Verification items for the finished model (mm, model axes). Give positions to 0.01 mm unless a question says otherwise; leave off trailing zeros. Loops run counter-clockwise (first coordinate to the right, second up) from the corner with the lowest first, then second, coordinate; pieces in that order, holes last. Notation, with made-up numbers: (83.5, -1) -> (91.5, -1) arc R11 ccw to (91.5, 17) -> close; hole circle Ø6 at (-17.5, -33). An arc over 180 degrees is marked (long way). Answer in a Markdown table with one row per item. Add a question column.
Q1. Gauge pin test, flat ends, axial feed: P1, Ø1, axis at x = -84.5, z = 151, coming from the +Y side; P2, Ø8, axis at x = -62.5, y = 32, coming from the -Z side. Record the tip position at first contact, or that the pin passes through.
Q2. Section check C-C on y = 187.5. Give the number of separate pieces and of enclosed holes in the cut face, and give its area (3 significant figures).
Q3. Section check A-A on x = -79.5. Enter the section's corners in (y, z).
Q4. Release check for a two-part mould opening along Z. For faces 1 (the face through (-2, 6.35, 88)), 2 (the face through (2, -6.35, 88)), 3 (the face through (1, 69, 0)) record: pulls with the +Z half, pulls with the -Z half, needs draft (parallel to the pull), parting line crosses it, or undercut.
Q5. Section check B-B on z = 105.5. Enter the section's corners in (x, y), and give its area (3 significant figures).
Q6. Material ranges on probe 1 along Y at (x, z) = (0, 173); probe 2 along Z at (x, y) = (1.5, 133); probe 3 along Y at (x, z) = (38.5, 35.5), recorded low to high.
```python
from build123d import *

# Parameters (mm, degrees)
SKETCH2_W           = 38.1
SKETCH2_H           = 12.7
BOSS_EXTRUDE1_DEPTH = 12.7
SKETCH4_W           = 228.702019181
SKETCH4_H           = 12.7
BOSS_EXTRUDE2_DEPTH = 152.4
SKETCH5_R           = 25.4
BOSS_EXTRUDE3_DEPTH = 12.7


with BuildPart() as part:
    # Sketch2 → Boss-Extrude1 (new body)
    with BuildSketch(Plane.XY):
        with BuildLine():
            add(Edge.make_bspline(
                [(-76.2, 6.35), (-38.1, 222.25), (0, 222.25)],
                knots=[0, 0, 0, 0.5, 0.5, 0.5], degree=2))
            Line((-76.2, 6.35), (-50.8, 6.35))
            Line((-50.8, 6.35), (0, 6.35))
            Line((0, 6.35), (0, 19.05))
            Line((0, 19.05), (0, 146.05))
            ThreePointArc((0, 146.05), (-25.4, 171.45), (0, 196.85))
            Line((0, 196.85), (0, 222.25))
        make_face()
        with BuildLine():
            add(Edge.make_bspline(
                [(-76.2, 6.35), (-38.1, 222.25), (0, 222.25)],
                knots=[0, 0, 0, 0.5, 0.5, 0.5], degree=2))
            Line((-76.2, 6.35), (-50.8, 6.35))
            Line((-50.8, 6.35), (0, 6.35))
            Line((0, 6.35), (0, 19.05))
            Line((0, 19.05), (0, 146.05))
            ThreePointArc((0, 146.05), (-25.4, 171.45), (0, 196.85))
            Line((0, 196.85), (0, 222.25))
        make_face()
        with BuildLine():
            add(Edge.make_bspline(
                [(0, 222.25), (38.1, 222.25), (76.2, 6.35)],
                knots=[0.5, 0.5, 0.5, 1, 1, 1], degree=2))
            Line((0, 222.25), (0, 196.85))
            ThreePointArc((0, 196.85), (17.960512242, 189.410512242), (25.4, 171.45))
            ThreePointArc((25.4, 171.45), (17.960512242, 153.489487758), (0, 146.05))
            Line((0, 146.05), (0, 19.05))
            Line((0, 19.05), (0, 6.35))
            Line((0, 6.35), (50.8, 6.35))
            Line((50.8, 6.35), (76.2, 6.35))
        make_face()
        with Locations((-95.25, 0)):
            Rectangle(SKETCH2_W, SKETCH2_H)
        Polygon((-50.8, 6.35), (-76.2, 6.35), (-76.2, -6.35), (76.2, -6.35), (76.2, 6.35), (50.8, 6.35), (0, 6.35), align=None)
        with Locations((95.25, 0)):
            Rectangle(SKETCH2_W, SKETCH2_H)
    extrude(amount=BOSS_EXTRUDE1_DEPTH)

    # Sketch4 → Boss-Extrude2 (add)
    with BuildSketch(Plane.XY.offset(12.7)):
        with Locations((0.051009591, 0)):
            Rectangle(SKETCH4_W, SKETCH4_H)
    extrude(amount=BOSS_EXTRUDE2_DEPTH)

    # Sketch5 → Boss-Extrude3 (add)
    with BuildSketch(Plane.XY.offset(165.1)):
        with BuildLine():
            Line((76.2, 6.35), (114.402019181, 6.35))
            Line((114.402019181, 6.35), (114.402019181, -6.35))
            Line((114.402019181, -6.35), (-114.3, -6.35))
            Line((-114.3, -6.35), (-114.3, 6.35))
            Line((-114.3, 6.35), (-76.2, 6.35))
            add(Edge.make_bspline(
                [(-76.2, 6.35), (0, 438.15), (76.2, 6.35)],
                knots=[0, 0, 0, 1, 1, 1], degree=2))
        make_face()
        with Locations((0, 171.45)):
            Circle(SKETCH5_R, mode=Mode.SUBTRACT)
    extrude(amount=BOSS_EXTRUDE3_DEPTH)


solid = part.part
```
Taken from the geometry:
| question | item | result |
|---|---|---|
| 1 | P1 | stops at y = 6.35 |
| 1 | P2 | stops at z = 0 |
| 2 | separate pieces | 4 |
| 2 | enclosed holes | 0 |
| 2 | area | 553 mm² |
| 3 | outline | (-6.35, 0) -> (6.35, 0) -> (6.35, 177.8) -> (-6.35, 177.8) -> close |
| 4 | face 1 | undercut |
| 4 | face 2 | needs draft |
| 4 | face 3 | pulls with the -Z half |
| 5 | outline | (-114.3, -6.35) -> (114.4, -6.35) -> (114.4, 6.35) -> (-114.3, 6.35) -> close |
| 5 | area | 2,900 mm² |
| 6 | probe 1 | y = -6.35 to 146.05, 196.85 to 222.25 |
| 6 | probe 2 | z = 0 to 12.7, 165.1 to 177.8 |
| 6 | probe 3 | y = -6.35 to 6.35 |
